Can you work these out from the drawing? Everything is in mm from the part's minimum corner. Give positions to 0.01 mm unless a question says otherwise; leave off trailing zeros. Order: outer loops, then holes, each group sorted by start corner. A loop starts at its lowest first (then second) coordinate and runs counter-clockwise, first axis right, second up. Notation, with made-up numbers: M 28.25,36 L 66.25,36 A25 cw 66.25,50 Z; hole C 74,2 d4. An arc over 180 degrees is marked long. Use a Markdown table: item, result. Add a question column.
Item 1: Suppose I cut it at C-C on x = 7.5. Write out the boundary of the cut face in (y, z).
Item 2: Suppose I cut it at A-A on z = 5. Write out the boundary of the cut face in (x, y), plus the area to 3 significant figures.
Item 3: Suppose I cut it at D-D on z = 7.75. Write out the boundary of the cut face in (x, y).
Item 4: If I drill on L1, parallel to X at y = 1.4, z = 5; L2, parallel to Z at x = 7.5, y = 1.95; L3, parallel to Z at x = 9, y = 3.2, over which ranges is the centre line in solid material (lowest first)? Write a range as from..to.
Item 5: If we mould it in two halves opening along X, with no side actions, what happens to the marked faces 1, 2 and 3? For each: released by +X, released by -X, zero draft, split by the parting line, or undercut.
Item 6: Suppose I cut it at B-B on y = 1.6. Write out the boundary of the cut face in (x, z), plus the area to 3 significant figures.
Item 7: I'm going to push flat-ended pins straight in: pin 1 Ø5 at (x, z) = (10, 1) entering from -Y; pin 2 Ø3 at (x, z) = (7.5, 5) entering from +Y (3 decimals). Where does each tip first touch, or does it pass through?
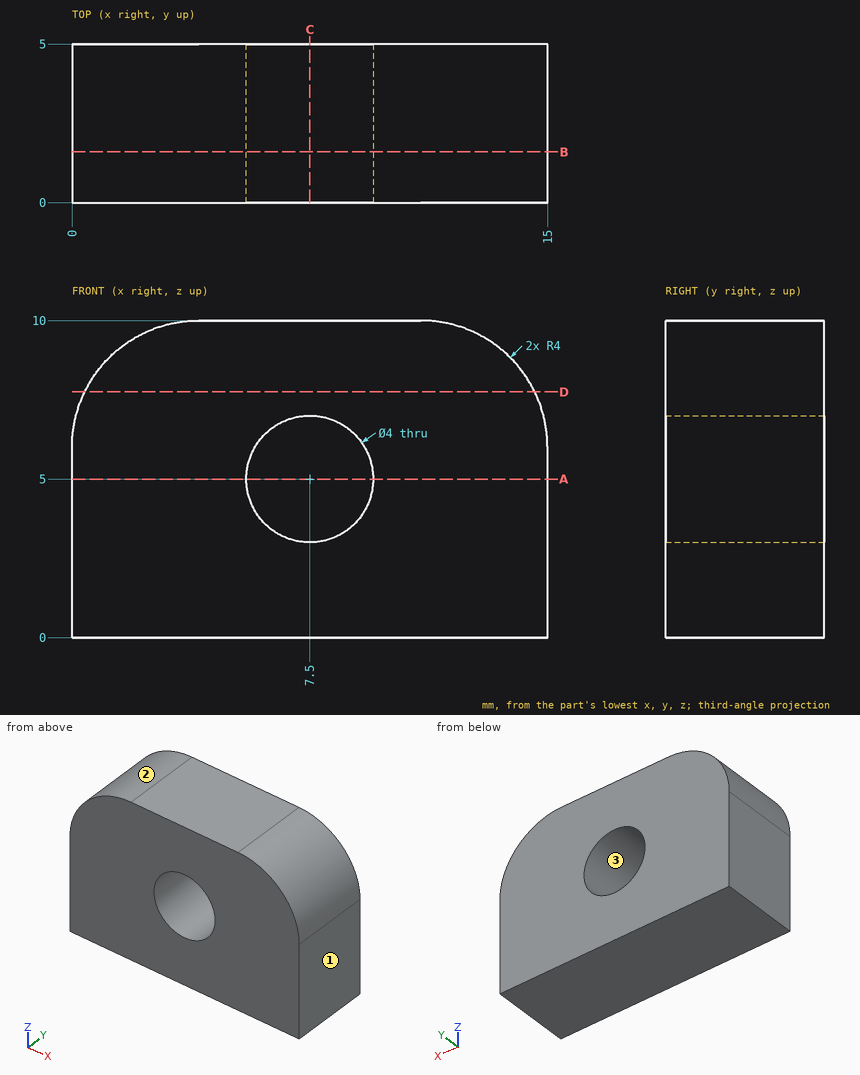
Findings below:
| question | item | result |
|---|---|---|
| 1 | outline | M 0,0 L 5,0 L 5,3 L 0,3 Z; M 0,7 L 5,7 L 5,10 L 0,10 Z |
| 2 | outline | M 0,0 L 5.5,0 L 5.5,5 L 0,5 Z; M 9.5,0 L 15,0 L 15,5 L 9.5,5 Z |
| 2 | area | 55.0 mm^2 |
| 3 | outline | M 0.4,0 L 14.6,0 L 14.6,5 L 0.4,5 Z |
| 4 | L1 | x = 0..5.5, 9.5..15 |
| 4 | L2 | z = 0..3, 7..10 |
| 4 | L3 | z = 0..3.68, 6.32..10 |
| 5 | face 1 | released by +X |
| 5 | face 2 | released by -X |
| 5 | face 3 | undercut |
| 6 | outline | M 0,0 L 15,0 L 15,6 A4 ccw 11,10 L 4,10 A4 ccw 0,6 Z; hole C 7.5,5 d4 |
| 6 | area | 131 mm^2 |
| 7 | pin 1 | stops at y = 0 |
| 7 | pin 2 | passes through |
